from build123d import *

# Parameters (mm, degrees)
SKETCH8_W                = 469.9
SKETCH8_H                = 419.1
BOSS_EXTRUDE1_DEPTH      = 50.8
CUT_EXTRUDE3_DEPTH       = 48.26
CUT_EXTRUDE4_DEPTH       = 48.26
CUT_EXTRUDE5_DEPTH       = 48.26
CUT_EXTRUDE6_DEPTH       = 48.26
CUT_EXTRUDE7_DEPTH       = 416.052
CUT_EXTRUDE8_DEPTH       = 69.342
CUT_EXTRUDE9_DEPTH       = 104.902
CUT_EXTRUDE9_DEPTH_BACK  = 516.128
CUT_EXTRUDE10_DEPTH      = 483.87
CUT_EXTRUDE10_DEPTH_BACK = 154.432
CUT_EXTRUDE11_DEPTH      = 419.608
CUT_EXTRUDE11_DEPTH_BACK = 113.03
FILLET1_R                = 50.8
FILLET2_R                = 50.8
FILLET3_R                = 50.8
FILLET4_R                = 50.8
CUT_EXTRUDE12_DEPTH      = 113.03
CUT_EXTRUDE13_DEPTH      = 113.03
CUT_EXTRUDE14_DEPTH      = 113.03
CUT_EXTRUDE15_DEPTH      = 113.03
CUT_EXTRUDE18_DEPTH      = 48.26
CUT_EXTRUDE18_TAPER      = 14
BODY_MOVE_COPY1_ANGLE    = 180


with BuildPart() as part:
    # Sketch8 → Boss-Extrude1 (new body)
    with BuildSketch(Plane(origin=(0, 0, 0), x_dir=(1, 0, 0), z_dir=(0, 1, 0))):
        with Locations((163.124113973, 170.845238095)):
            Rectangle(SKETCH8_W, SKETCH8_H)
    extrude(amount=-BOSS_EXTRUDE1_DEPTH)

    # Sketch9 → Cut-Extrude3 (cut)
    with BuildSketch(Plane(origin=(0, 0, 0), x_dir=(1, 0, 0), z_dir=(0, 1, 0))):
        Polygon((-46.425886027, -13.304761905), (372.674113973, -13.304761905), (398.074113973, -38.704761905), (-71.825886027, -38.704761905), align=None)
    extrude(amount=-CUT_EXTRUDE3_DEPTH, mode=Mode.SUBTRACT)

    # Sketch11 → Cut-Extrude4 (cut)
    with BuildSketch(Plane(origin=(0, 0, 0), x_dir=(1, 0, 0), z_dir=(0, 1, 0))):
        Polygon((-46.425886027, 354.995238095), (-46.425886027, -13.304761905), (-71.825886027, -38.704761905), (-71.825886027, 380.395238095), align=None)
    extrude(amount=-CUT_EXTRUDE4_DEPTH, mode=Mode.SUBTRACT)

    # Sketch13 → Cut-Extrude5 (cut)
    with BuildSketch(Plane(origin=(0, 0, 0), x_dir=(1, 0, 0), z_dir=(0, 1, 0))):
        Polygon((-46.425886027, 354.995238095), (372.674113973, 354.995238095), (398.074113973, 380.395238095), (-71.825886027, 380.395238095), align=None)
    extrude(amount=-CUT_EXTRUDE5_DEPTH, mode=Mode.SUBTRACT)

    # Sketch14 → Cut-Extrude6 (cut)
    with BuildSketch(Plane(origin=(0, 0, 0), x_dir=(1, 0, 0), z_dir=(0, 1, 0))):
        Polygon((398.074113973, 380.395238095), (372.674113973, 354.995238095), (372.674113973, -13.304761905), (398.074113973, -38.704761905), align=None)
    extrude(amount=-CUT_EXTRUDE6_DEPTH, mode=Mode.SUBTRACT)

    # Sketch16 → Cut-Extrude7 (cut)
    with BuildSketch(Plane.XY):
        Polygon((-46.425886027, 0), (-33.725886027, 0), (-46.425886027, -48.26), align=None)
    extrude(amount=-CUT_EXTRUDE7_DEPTH, mode=Mode.SUBTRACT)

    # Sketch17 → Cut-Extrude8 (cut)
    with BuildSketch(Plane.XY):
        Polygon((-33.725886027, 0), (-46.425886027, 0), (-46.425886027, -48.26), align=None)
    extrude(amount=CUT_EXTRUDE8_DEPTH, mode=Mode.SUBTRACT)

    # Sketch18 → Cut-Extrude9 (cut, two sides: drawn at the far end of the back side and taken through both)
    with BuildSketch(Plane.XY.offset(-CUT_EXTRUDE9_DEPTH_BACK)):
        Polygon((372.674113973, 0), (359.974113973, 0), (372.674113973, -48.26), align=None)
    extrude(amount=CUT_EXTRUDE9_DEPTH + CUT_EXTRUDE9_DEPTH_BACK, mode=Mode.SUBTRACT)

    # Sketch19 → Cut-Extrude10 (cut, two sides: drawn at the far end of the back side and taken through both)
    with BuildSketch(Plane(origin=(0, 0, 0), x_dir=(0, 0, -1), z_dir=(1, 0, 0)).offset(-CUT_EXTRUDE10_DEPTH_BACK)):
        Polygon((-13.304761905, 0), (-0.604761905, 0), (-13.304761905, -48.26), align=None)
    extrude(amount=CUT_EXTRUDE10_DEPTH + CUT_EXTRUDE10_DEPTH_BACK, mode=Mode.SUBTRACT)

    # Sketch20 → Cut-Extrude11 (cut, two sides: drawn at the far end of the back side and taken through both)
    with BuildSketch(Plane(origin=(0, 0, 0), x_dir=(0, 0, -1), z_dir=(1, 0, 0)).offset(-CUT_EXTRUDE11_DEPTH_BACK)):
        Polygon((354.995238095, 0), (342.295238095, 0), (354.995238095, -48.26), align=None)
    extrude(amount=CUT_EXTRUDE11_DEPTH + CUT_EXTRUDE11_DEPTH_BACK, mode=Mode.SUBTRACT)

    # Fillet1
    fillet1_edges = [part.edges().sort_by_distance(p)[0] for p in [
        (-40.075886027, -24.13, 6.954761905),
    ]]
    fillet(fillet1_edges, radius=FILLET1_R)

    # Fillet2
    fillet2_edges = [part.edges().sort_by_distance(p)[0] for p in [
        (-40.075886027, -24.13, -348.645238095),
    ]]
    fillet(fillet2_edges, radius=FILLET2_R)

    # Fillet3
    fillet3_edges = [part.edges().sort_by_distance(p)[0] for p in [
        (366.324113973, -24.13, -348.645238095),
    ]]
    fillet(fillet3_edges, radius=FILLET3_R)

    # Fillet4
    fillet4_edges = [part.edges().sort_by_distance(p)[0] for p in [
        (366.324113973, -24.13, 6.954761905),
    ]]
    fillet(fillet4_edges, radius=FILLET4_R)

    # Sketch24 → Cut-Extrude12 (cut)
    with BuildSketch(Plane(origin=(0, 0, 0), x_dir=(1, 0, 0), z_dir=(0, 1, 0))):
        with BuildLine():
            Line((-71.825886027, -38.704761905), (-21.025886027, -38.704761905))
            ThreePointArc((-21.025886027, -38.704761905), (-56.946910511, -23.825786389), (-71.825886027, 12.095238095))
            Line((-71.825886027, 12.095238095), (-71.825886027, -38.704761905))
        make_face()
    extrude(amount=-CUT_EXTRUDE12_DEPTH, mode=Mode.SUBTRACT)

    # Sketch25 → Cut-Extrude13 (cut)
    with BuildSketch(Plane(origin=(0, 0, 0), x_dir=(1, 0, 0), z_dir=(0, 1, 0))):
        with BuildLine():
            Line((-71.825886027, 380.395238095), (-21.025886027, 380.395238095))
            ThreePointArc((-21.025886027, 380.395238095), (-56.946910511, 365.51626258), (-71.825886027, 329.595238095))
            Line((-71.825886027, 329.595238095), (-71.825886027, 380.395238095))
        make_face()
    extrude(amount=-CUT_EXTRUDE13_DEPTH, mode=Mode.SUBTRACT)

    # Sketch26 → Cut-Extrude14 (cut)
    with BuildSketch(Plane(origin=(0, 0, 0), x_dir=(1, 0, 0), z_dir=(0, 1, 0))):
        with BuildLine():
            Line((398.074113973, 380.395238095), (347.274113973, 380.395238095))
            ThreePointArc((347.274113973, 380.395238095), (383.195138458, 365.51626258), (398.074113973, 329.595238095))
            Line((398.074113973, 329.595238095), (398.074113973, 380.395238095))
        make_face()
    extrude(amount=-CUT_EXTRUDE14_DEPTH, mode=Mode.SUBTRACT)

    # Sketch27 → Cut-Extrude15 (cut)
    with BuildSketch(Plane(origin=(0, 0, 0), x_dir=(1, 0, 0), z_dir=(0, 1, 0))):
        with BuildLine():
            Line((398.074113973, -38.704761905), (347.274113973, -38.704761905))
            ThreePointArc((347.274113973, -38.704761905), (383.195138458, -23.825786389), (398.074113973, 12.095238095))
            Line((398.074113973, 12.095238095), (398.074113973, -38.704761905))
        make_face()
    extrude(amount=-CUT_EXTRUDE15_DEPTH, mode=Mode.SUBTRACT)

    # Sketch29 → Cut-Extrude18 (cut)
    with BuildSketch(Plane(origin=(0, -50.8, 0), x_dir=(1, 0, 0), z_dir=(0, 1, 0))):
        with BuildLine():
            ThreePointArc((310.846727481, 12.095238095), (336.604779491, 22.764572578), (347.274113973, 48.522624588))
            Line((347.274113973, 48.522624588), (347.274113973, 293.167851602))
            ThreePointArc((347.274113973, 293.167851602), (336.604779491, 318.925903612), (310.846727481, 329.595238095))
            Line((310.846727481, 329.595238095), (15.401500466, 329.595238095))
            ThreePointArc((15.401500466, 329.595238095), (-10.356551544, 318.925903612), (-21.025886027, 293.167851602))
            Line((-21.025886027, 293.167851602), (-21.025886027, 48.522624588))
            ThreePointArc((-21.025886027, 48.522624588), (-10.356551544, 22.764572578), (15.401500466, 12.095238095))
            Line((15.401500466, 12.095238095), (310.846727481, 12.095238095))
        make_face()
    extrude(amount=CUT_EXTRUDE18_DEPTH, taper=CUT_EXTRUDE18_TAPER, mode=Mode.SUBTRACT)


with BuildPart() as part_1:
    # Body-Move/Copy1: moved
    add(part.part.rotate(Axis((163.124113973, -25.4, 0), (0, 0, 1)), BODY_MOVE_COPY1_ANGLE))


solid = part_1.part
Source: CAD feature listing. Evaluate the final solid. Frame: model axes, mm. A direction names the side the tool comes from. Coordinates: 2 decimals unless noted, no trailing zeros. Answer in a Markdown table with one row per item. Add a question column.
Q1. Pull-direction query (Z, two-part tool) for faces 1 (the face through (166, -50.8, -173)), 2 (the face through (-25.66, -28.915, -8.218)), 3 (the face through (332.05, -24.47, -314.85)); classes: pulls with the +Z half, pulls with the -Z half, needs draft (parallel to the pull), parting line crosses it, or undercut.
Q2. Ray query, line 1 along Y through (x, z) = (294, -165); line 2 along Z through (x, y) = (273.5, -23.5); line 3 along Z through (x, y) = (203.5, -13). Return the intervals inside material, ascending.
Q3. Contact query for flat-ended pins moving along their axis: pin 1 Ø12 at (x, y) = (124, -9.5) entering from -Z; pin 2 Ø10 at (x, y) = (72.5, -45) entering from +Z; pin 3 Ø3 at (y, z) = (-13.5, -327.5) entering from -X; pin 4 Ø10 at (x, y) = (-21.5, -5) entering from -Z. Output: stop coordinate, or through.
Q4. Reachability of faces 4 (the face through (182, -2.54, 14)), 5 (the face through (332.5, -24.5, -27.3)), 6 (the face through (366.235, -27.008, -168.955)) from +Z, -Z, +X, -X, +Y, -Y: full face, straight path, thin tool, end or side. Return the list, or none.
Computed values:
| question | item | result |
|---|---|---|
| 1 | face 1 | needs draft |
| 1 | face 2 | pulls with the +Z half |
| 1 | face 3 | undercut |
| 2 | line 1 | y = -50.8 to -48.26 |
| 2 | line 2 | z = -349.48 to -323.74, -17.95 to 7.79 |
| 2 | line 3 | z = -352.24 to -326.35, -15.34 to 10.55 |
| 3 | pin 1 | stops at z = -354.74 |
| 3 | pin 2 | stops at z = 3.45 |
| 3 | pin 3 | stops at x = -38.23 |
| 3 | pin 4 | stops at z = -380.4 |
| 4 | face 4 | -Y |
| 4 | face 5 | +Y |
| 4 | face 6 | +Z, -Z, +X, -Y |
